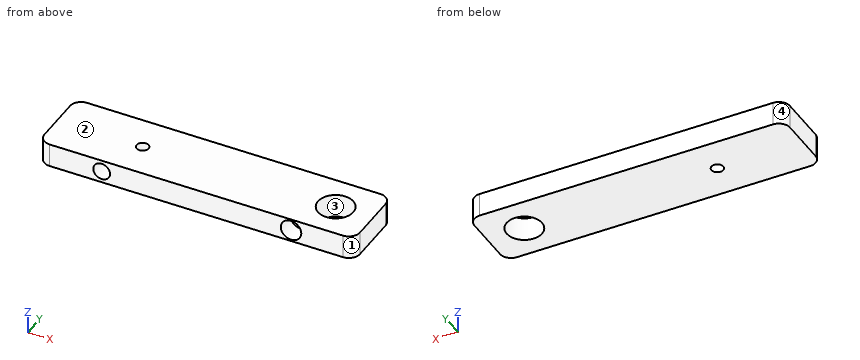
```python
from build123d import *

# Parameters (mm, degrees)
F0_W     = 85
F0_H     = 19.05
F0_R     = 1.6
F0_R_2   = 4.75
F1_DEPTH = 3.175
F2_R     = 2.249345
F2_R_2   = 2.765541
F3_DEPTH = 5
F4_R     = 3


with BuildPart() as f1:
    # F0 (on Top) → F1 (new body, symmetric)
    with BuildSketch(Plane.XY):
        Rectangle(F0_W, F0_H)
        with Locations((-19.5, 0)):
            Circle(F0_R, mode=Mode.SUBTRACT)
        with Locations((32.5, 0)):
            Circle(F0_R_2, mode=Mode.SUBTRACT)
    extrude(amount=F1_DEPTH, both=True)

    # F2 (on face) → F3 (cut)
    with BuildSketch(Plane.XZ.offset(9.525)):
        with Locations((-25.5, 0)):
            Circle(F2_R)
        with Locations((25.5, 0)):
            Circle(F2_R_2)
    extrude(amount=-F3_DEPTH, mode=Mode.SUBTRACT)

    # F4
    f4_edges = [f1.edges().sort_by_distance(p)[0] for p in [
        (42.5, -9.525, 0),
        (42.5, 9.525, 0),
        (-42.5, -9.525, 0),
        (-42.5, 9.525, 0),
    ]]
    fillet(f4_edges, radius=F4_R)


solid = f1.part
```
Verification items for the finished model (mm, model axes). Face numbers are marked on the shaded views. Coordinates: 2 decimals unless noted, no trailing zeros. Loops run counter-clockwise (first coordinate to the right, second up) from the corner with the lowest first, then second, coordinate; pieces in that order, holes last. Notation, with made-up numbers: (5, -6.5) - (18, -6.5) arc R21 cw to (18, 31.5) - close; hole circle Ø3 at (-36, -22.75). An arc over 180 degrees is marked (long way). Return JSON: item names as keys, results as strings.
1. Section check D-D, the plane x = 25.5. Record the boundary of the cut face in (y, z) (3 decimals), then the cut area to 3 significant figures.
Established:
{"outline": "(-9.525, -3.175) - (9.525, -3.175) - (9.525, 3.175) - (-9.525, 3.175) - (-9.525, 2.766) - (-4.525, 2.766) - (-4.525, -2.766) - (-9.525, -2.766) - close", "area": "93.3 mm2"}
2. Mould release check, pull along Y, two halves, no side actions. Record for the marked faces 1, 2, 3 and 4: +Y half, -Y half, draft (parallel to the pull), parting line (faces both ways), or undercut.
Established:
{"face 1": "-Y half", "face 2": "draft", "face 3": "undercut", "face 4": "+Y half"}
3. Section check A-A, the plane x = -19.5. Record the boundary of the cut face in (y, z) (3 decimals), then the cut area to 3 significant figures.
Established:
{"outline": "(-9.525, -3.175) - (-1.6, -3.175) - (-1.6, 3.175) - (-9.525, 3.175) - close; (1.6, -3.175) - (9.525, -3.175) - (9.525, 3.175) - (1.6, 3.175) - close", "area": "101 mm2"}
4. Thickness scan on L1, parallel to Y at x = 32.5, z = 2.25 (3 decimals); L2, parallel to X at y = -6.75, z = 1.5; L3, parallel to Z at x = -25.5, y = -7.7 (3 decimals). Record the ranges inside material, lowest first.
Established:
{"L1": "y = -9.525 to -4.75, 4.75 to 9.525", "L2": "x = -42.49 to -27.18, -23.82 to 23.18, 27.82 to 42.49", "L3": "z = -3.175 to -2.249, 2.249 to 3.175"}
5. Section check B-B, the plane y = 0. Record the boundary of the cut face in (x, z) (3 decimals).
Established:
{"outline": "(-42.5, -3.175) - (-21.1, -3.175) - (-21.1, 3.175) - (-42.5, 3.175) - close; (-17.9, -3.175) - (27.75, -3.175) - (27.75, 3.175) - (-17.9, 3.175) - close; (37.25, -3.175) - (42.5, -3.175) - (42.5, 3.175) - (37.25, 3.175) - close"}
6. Go/stop test with flat-tipped pins: pin 1 (1.7 mm diameter, centred on x = 25.5, z = 0, fed in from -Y) (3 decimals); pin 2 (1.5 mm diameter, centred on y = 7.5, z = -2, fed in from -X); pin 3 (11 mm diameter, centred on x = 32.5, y = 0, fed in from +Z) (3 decimals). Record where each tip stops, or that it passes through.
Established:
{"pin 1": "stops at y = -4.525", "pin 2": "stops at x = -42.49", "pin 3": "stops at z = 3.175"}
7. Section check C-C, the plane z = 0. Record the boundary of the cut face in (x, y) (3 decimals), then the cut area to 3 significant figures.
Established:
{"outline": "(-42.5, -6.525) arc R3 ccw to (-39.5, -9.525) - (-27.749, -9.525) - (-27.749, -4.525) - (-23.251, -4.525) - (-23.251, -9.525) - (22.734, -9.525) - (22.734, -4.525) - (28.266, -4.525) - (28.266, -9.525) - (39.5, -9.525) arc R3 ccw to (42.5, -6.525) - (42.5, 6.525) arc R3 ccw to (39.5, 9.525) - (-39.5, 9.525) arc R3 ccw to (-42.5, 6.525) - close; hole circle Ø3.2 at (-19.5, 0); hole circle Ø9.5 at (32.5, 0)", "area": "1,480 mm2"}
